Build history of the part. All positions in model axes, mm. Round coordinates to 2 decimals unless told otherwise and drop trailing zeros. Loops run counter-clockwise (first coordinate to the right, second up) from the corner with the lowest first, then second, coordinate; pieces in that order, holes last. Notation, with made-up numbers: (-16.5, -25.5) - (26.5, -25.5) arc R28 cw to (26.5, -5.5) - close; hole circle Ø1 at (-9.5, 61.5). An arc over 180 degrees is marked (long way). Use a Markdown table: item, result.
from build123d import *

# Parameters (mm, degrees)
SKETCH1_R     = 2
SKETCH1_R_2   = 1.3
CHAMFER1_SIZE = 0.127


with BuildPart() as part:
    # Sweep1: sweep along a curve in space
    with BuildLine() as sweep1_path:
        Line((-150.085279081, -93.282256564, 25.525), (-150.085279081, -103.482256564, 25.525))
        add(Edge.make_bspline(
            [(-143.943719565, -46.6, 27.001622999), (-143.943719565, -51.770788857, 27.001622999), (-147.014499323, -75.131743905, 26.263311499), (-150.085279081, -82.551529797, 25.525), (-150.085279081, -93.282256564, 25.525)],
            knots=[0, 0, 0, 0, 0.329296004, 1, 1, 1, 1], degree=3))
        Line((-143.943719565, -35.8, 27.001622999), (-143.943719565, -46.6, 27.001622999))
    # Sketch1 → Sweep1 (sweep)
    with BuildSketch(Plane(origin=(0, -95.382256564, 0), x_dir=(1, 0, 0), z_dir=(0, 1, 0))):
        with Locations((-150.085279081, -25.525)):
            Circle(SKETCH1_R)
        with Locations((-150.085279081, -25.525)):
            Circle(SKETCH1_R_2, mode=Mode.SUBTRACT)
    sweep(path=sweep1_path.line)

    # Chamfer1
    chamfer1_edges = [part.edges().sort_by_distance(p)[0] for p in [
        (-145.243719565, -35.8, 27.001622999),
        (-145.943719565, -35.8, 27.001622999),
        (-151.385279081, -103.482256564, 25.525),
        (-152.085279081, -103.482256564, 25.525),
    ]]
    chamfer(chamfer1_edges, length=CHAMFER1_SIZE)


solid = part.part
Q1. Pull direction Z, two halves, no side cores. Call faces 1 (the face through (-151.384, -98.389, 25.582)), 2 (the face through (-148.238, -98.389, 24.759)): pulls with the +Z half, pulls with the -Z half, needs draft (parallel to the pull), parting line crosses it, or undercut.
Results found:
| item | result |
|---|---|
| face 1 | undercut |
| face 2 | parting line crosses it |
Q2. Probe line 1 (X direction, y = -39.5, z = 27.4); line 2 (Z direction, x = -145.75, y = -70); line 3 (X direction, y = -48, z = 26.2). List the from-to ranges inside material, lowest first.
Results found:
| item | result |
|---|---|
| line 1 | x = -145.9 to -145.18, -142.71 to -141.98 |
| line 2 | z = 24.61 to 25.53, 27.12 to 28.04 |
| line 3 | x = -145.8 to -144.99, -142.94 to -142.13 |
Q3. Drop flat-ended pins along their axis: pin 1 (5 mm diameter, centred on x = -145, y = -57, fed in from +Z); pin 2 (1.5 mm diameter, centred on y = -69, z = 26, fed in from +X); pin 3 (3 mm diameter, centred on x = -149, y = -82, fed in from +Z); pin 4 (2 mm diameter, centred on x = -145, y = -86.5, fed in from -Z). Give the stop position or say it passes through.
Results found:
| item | result |
|---|---|
| pin 1 | stops at z = 28.88 |
| pin 2 | stops at x = -144.45 |
| pin 3 | stops at z = 27.81 |
| pin 4 | passes through |
Q4. Cut at A-A, the plane y = -98. List the corners of the cut face in (x, z) (3 decimals).
Results found:
| item | result |
|---|---|
| outline | circle Ø4 at (-150.085, 25.525); hole circle Ø2.6 at (-150.085, 25.525) |
